from build123d import *

# Parameters (mm, degrees)
F0_W      = 8.235
F0_H      = 90.17
F0_W_2    = 79.38
F0_H_2    = 12.7
F1_DEPTH  = 1.73
F2_W      = 8.13
F2_H      = 65.02
F3_DEPTH  = 10.42
F4_W      = 2.38
F4_H      = 13.8
F4_H_2    = 7.45
F4_W_2    = 65.44
F4_H_3    = 17.54
F5_DEPTH  = 5.18
F6_W      = 9.3
F6_H      = 30
F7_DEPTH  = 5.58
F8_W      = 73.03
F8_H      = 90.17
F9_DEPTH  = 25.4
F10_W     = 11.41
F10_H     = 8.13
F10_H_2   = 10.54
F10_H_3   = 11.81
F11_DEPTH = 11.1
F12_W     = 75.51
F12_H     = 5.75
F13_DEPTH = 6.43
F14_W     = 5.72
F14_H     = 61.39
F15_DEPTH = 5.57
F16_W     = 77.07
F16_H     = 5.75
F17_DEPTH = 6.43
F18_W     = 6.17
F18_H     = 46.82
F19_DEPTH = 6.43
F20_W     = 9.78
F20_H     = 18.65
F21_DEPTH = 7.35
F22_R     = 1.6
F23_DEPTH = 27.131


with BuildPart() as f1:
    # F0 (on Top) → F1 (new body)
    with BuildSketch(Plane.XY):
        with Locations((43.8075, 0)):
            Rectangle(F0_W, F0_H)
        with Locations((0, -51.435)):
            Rectangle(F0_W_2, F0_H_2)
        Rectangle(F0_W_2, F0_H)
        with Locations((-43.8075, 0)):
            Rectangle(F0_W, F0_H)
        with Locations((0, 51.435)):
            Rectangle(F0_W_2, F0_H_2)
    extrude(amount=F1_DEPTH)

    # F2 (on face) → F3 (join)
    with BuildSketch(Plane(origin=(0, 0, 0), x_dir=(1, 0, 0), z_dir=(0, 0, -1))):
        with Locations((40.56, -0.075)):
            Rectangle(F2_W, F2_H)
    extrude(amount=F3_DEPTH)

    # F4 (on face) → F5 (join)
    with BuildSketch(Plane(origin=(0, 0, 0), x_dir=(1, 0, 0), z_dir=(0, 0, -1))):
        with Locations((-36.21, -39.8490008428)):
            Rectangle(F4_W, F4_H)
        with Locations((-36.21, -50.4740008428)):
            Rectangle(F4_W, F4_H_2)
        with Locations((-2.3, -50.4740008428)):
            Rectangle(F4_W_2, F4_H_2)
        with Locations((31.61, -37.9790008428)):
            Rectangle(F4_W, F4_H_3)
        with Locations((31.61, -50.4740008428)):
            Rectangle(F4_W, F4_H_2)
    extrude(amount=F5_DEPTH)

    # F6 (on face) → F7 (join)
    with BuildSketch(Plane(origin=(0, 0, 0), x_dir=(1, 0, 0), z_dir=(0, 0, -1))):
        with Locations((-32.925, 31.505)):
            Rectangle(F6_W, F6_H)
    extrude(amount=F7_DEPTH)

    # F8 (on face) → F9 (join)
    with BuildSketch(Plane.XY.offset(1.73)):
        Rectangle(F8_W, F8_H)
    extrude(amount=F9_DEPTH)

    # F10 (on face) → F11 (join)
    with BuildSketch(Plane.XY.offset(1.73)):
        with Locations((42.22, 41.02)):
            Rectangle(F10_W, F10_H)
        with Locations((42.22, -41.02)):
            Rectangle(F10_W, F10_H)
        with Locations((-42.22, 39.815)):
            Rectangle(F10_W, F10_H_2)
        with Locations((-42.22, -39.18)):
            Rectangle(F10_W, F10_H_3)
    extrude(amount=F11_DEPTH)

    # F12 (on face) → F13 (join)
    with BuildSketch(Plane.XY.offset(1.73)):
        with Locations((-0.875, -52.63)):
            Rectangle(F12_W, F12_H)
    extrude(amount=F13_DEPTH)

    # F14 (on face) → F15 (join)
    with BuildSketch(Plane.XY.offset(1.73)):
        with Locations((-42.915, 3.25)):
            Rectangle(F14_W, F14_H)
    extrude(amount=F15_DEPTH)

    # F16 (on face) → F17 (join)
    with BuildSketch(Plane.XY.offset(1.73)):
        with Locations((-0.095, 52.67)):
            Rectangle(F16_W, F16_H)
    extrude(amount=F17_DEPTH)

    # F18 (on face) → F19 (join)
    with BuildSketch(Plane.XY.offset(1.73)):
        with Locations((42.56, -13.065)):
            Rectangle(F18_W, F18_H)
    extrude(amount=F19_DEPTH)

    # F20 (on face) → F21 (join)
    with BuildSketch(Plane.XY.offset(1.73)):
        with Locations((43.035, 24.36)):
            Rectangle(F20_W, F20_H)
    extrude(amount=F21_DEPTH)

    # F22 (on face) → F23 (cut, through all)
    with BuildSketch(Plane(origin=(0, 0, 0), x_dir=(1, 0, 0), z_dir=(0, 0, -1))):
        with Locations((42.845, 40.005)):
            Circle(F22_R)
        with Locations((42.845, -40.005)):
            Circle(F22_R)
        with Locations((-42.845, -37.455)):
            Circle(F22_R)
        with Locations((-42.845, 36.185)):
            Circle(F22_R)
    extrude(amount=-F23_DEPTH, mode=Mode.SUBTRACT)


solid = f1.part
CAD build for the part. Positions are in the model's coordinates, mm. A direction names the side the tool comes from. Coordinates: 2 decimals unless noted, no trailing zeros. Loops run counter-clockwise (first coordinate to the right, second up) from the corner with the lowest first, then second, coordinate; pieces in that order, holes last. Notation, with made-up numbers: (82, 37.25) -> (109, 37.25) arc R13 ccw to (109, 42.25) -> close; hole circle Ø1 at (72.5, 0). An arc over 180 degrees is marked (long way). One line per item, written item: value.
1. Flat gauge pins, fed straight in: P1, Ø5, axis at x = 37.5, z = -5, coming from the +Y side (3 decimals); P2, Ø1.7, axis at x = 2.5, y = 54, coming from the +Z side; P3, Ø8, axis at x = 22, z = 16.5, coming from the -Y side (3 decimals). Where does each tip first touch, or does it go through?
Answers:
P1: stops at y = 32.585
P2: stops at z = 8.16
P3: stops at y = -45.085
2. Which spindle directions (+Z, -Z, +X, -X, +Y, -Y) get a long thin tool onto all of the face, cutting with end or side? Do faces 1 (the face through (30.42, 38, -3)), 2 (the face through (36.495, 1, -5)), 3 (the face through (42, -36.955, 7)), 4 (the face through (38.145, 24, 5)). Say none if no direction does.
Answers:
face 1: -Z, -Y
face 2: -Z, +Y, -Y
face 3: +Z, +X
face 4: +Z
3. Drill centre lines: line 1 (X direction, y = -8.5, z = 3) (3 decimals); line 2 (Y direction, x = -17, z = 4) (3 decimals); line 3 (Y direction, x = 41, z = 9.5) (3 decimals). Where is each one in solid material? Low to high. Write a range as [from, to].
Answers:
line 1: x = [-45.775, -40.055], [-36.515, 36.515], [39.475, 45.645]
line 2: y = [-55.505, -49.755], [-45.085, 45.085], [49.795, 55.545]
line 3: y = [-45.085, -36.955], [36.955, 45.085]
4. Pull direction X, two halves, no side cores. Call faces 5 (the face through (-33, -46.505, -3)), 6 (the face through (36.515, -1, 14)), 7 (the face through (-38.63, -53, 5)), 8 (the face through (38.44, 53, 5)): pulls with the +X half, pulls with the -X half, needs draft (parallel to the pull), parting line crosses it, or undercut.
Answers:
face 5: needs draft
face 6: undercut
face 7: pulls with the -X half
face 8: pulls with the +X half
5. Slice it at D-D on y = -24.5. Write the cut outline in (x, z) (3 decimals), and give its area (3 significant figures).
Answers:
outline: (-47.925, 0) -> (-37.575, 0) -> (-37.575, -5.58) -> (-28.275, -5.58) -> (-28.275, 0) -> (36.495, 0) -> (36.495, -10.42) -> (44.625, -10.42) -> (44.625, 0) -> (47.925, 0) -> (47.925, 1.73) -> (45.645, 1.73) -> (45.645, 8.16) -> (39.475, 8.16) -> (39.475, 1.73) -> (36.515, 1.73) -> (36.515, 27.13) -> (-36.515, 27.13) -> (-36.515, 1.73) -> (-40.055, 1.73) -> (-40.055, 7.3) -> (-45.775, 7.3) -> (-45.775, 1.73) -> (-47.925, 1.73) -> close
area: 2,230 mm^2
6. Slice it at A-A on z = -2. Write the cut outline in (x, y) (3 decimals), and give its area (3 significant figures).
Answers:
outline: (-37.575, -46.505) -> (-28.275, -46.505) -> (-28.275, -16.505) -> (-37.575, -16.505) -> close; (-37.4, 32.949) -> (-35.02, 32.949) -> (-35.02, 46.749) -> (30.42, 46.749) -> (30.42, 29.209) -> (32.8, 29.209) -> (32.8, 54.199) -> (-37.4, 54.199) -> close; (36.495, -32.435) -> (44.625, -32.435) -> (44.625, 32.585) -> (36.495, 32.585) -> close
area: 1,410 mm^2
7. Slice it at C-C on x = 26.5. Write the cut outline in (y, z) (3 decimals), and give its area (3 significant figures).
Answers:
outline: (-57.785, 0) -> (46.749, 0) -> (46.749, -5.18) -> (54.199, -5.18) -> (54.199, 0) -> (57.785, 0) -> (57.785, 1.73) -> (55.545, 1.73) -> (55.545, 8.16) -> (49.795, 8.16) -> (49.795, 1.73) -> (45.085, 1.73) -> (45.085, 27.13) -> (-45.085, 27.13) -> (-45.085, 1.73) -> (-49.755, 1.73) -> (-49.755, 8.16) -> (-55.505, 8.16) -> (-55.505, 1.73) -> (-57.785, 1.73) -> close
area: 2,600 mm^2
8. Slice it at B-B on y = 19.5. Write the cut outline in (x, z) (3 decimals).
Answers:
outline: (-47.925, 0) -> (36.495, 0) -> (36.495, -10.42) -> (44.625, -10.42) -> (44.625, 0) -> (47.925, 0) -> (47.925, 9.08) -> (38.145, 9.08) -> (38.145, 1.73) -> (36.515, 1.73) -> (36.515, 27.13) -> (-36.515, 27.13) -> (-36.515, 1.73) -> (-40.055, 1.73) -> (-40.055, 7.3) -> (-45.775, 7.3) -> (-45.775, 1.73) -> (-47.925, 1.73) -> close
